Verification items for the finished model (mm, model axes). A direction names the side the tool comes from. Give positions to 0.01 mm unless a question says otherwise; leave off trailing zeros. Loops run counter-clockwise (first coordinate to the right, second up) from the corner with the lowest first, then second, coordinate; pieces in that order, holes last. Notation, with made-up numbers: M 15,73.5 L 53,73.5 A21 cw 53,112.5 Z; hole C -25.5,72.5 d10. An arc over 180 degrees is marked long. Put each result on its own line as item: value. Start each with the question number.
from build123d import *

# Parameters (mm, degrees)
SKETCH1_R           = 1.375
BOSS_EXTRUDE1_DEPTH = 6
BOSS_EXTRUDE2_START = -13.125
SKETCH9_W           = 3.5
SKETCH9_H           = 3
BOSS_EXTRUDE2_DEPTH = 7.26
BOSS_EXTRUDE3_START = -26.75
SKETCH10_W          = 3
SKETCH10_H          = 3
BOSS_EXTRUDE3_DEPTH = 23.25
SKETCH11_W          = 3
SKETCH11_H          = 3
BOSS_EXTRUDE4_DEPTH = 5
FILLET1_R           = 2.5
FILLET2_R           = 1


with BuildPart() as part:
    # Sketch1 → Boss-Extrude1 (new body)
    with BuildSketch(Plane(origin=(0, 0, 0), x_dir=(0, 1, 0), z_dir=(0, 0, 1))):
        with BuildLine():
            Line((0, 2.875), (7, 2.875))
            Line((7, 2.875), (7, -2.875))
            Line((7, -2.875), (0, -2.875))
            ThreePointArc((0, -2.875), (-2.875, 0), (0, 2.875))
        make_face()
        with Locations(Location((0, 0, 0), (0, 0, 270))):
            Circle(SKETCH1_R, mode=Mode.SUBTRACT)
    extrude(amount=BOSS_EXTRUDE1_DEPTH)

    # Sketch2 → Loft1 section 0
    with BuildSketch(Plane(origin=(0, 0, 0), x_dir=(1, 0, 0), z_dir=(0, 0, -1))):
        with BuildLine():
            Line((0.875, -7), (-2.875, -7))
            Line((-2.875, -7), (-2.875, -3.5))
            Line((-2.875, -3.5), (0.875, -3.5))
            Line((0.875, -3.5), (0.875, -7))
        make_face()
    # Sketch8 → Loft1 section 1
    with BuildSketch(Plane(origin=(0, 0, -37.5), x_dir=(-1, 0, 0), z_dir=(0, 0, -1))):
        with BuildLine():
            Line((2.375, 3.5), (2.375, 7))
            Line((2.375, 7), (6.125, 7))
            Line((6.125, 7), (6.125, 3.5))
            Line((6.125, 3.5), (2.375, 3.5))
        make_face()
    loft()

    # Sketch9 → Boss-Extrude2 (add)
    with BuildSketch(Plane.YZ.offset(BOSS_EXTRUDE2_START)):
        with Locations((5.25, -36)):
            Rectangle(SKETCH9_W, SKETCH9_H)
    extrude(amount=BOSS_EXTRUDE2_DEPTH)

    # Sketch10 → Boss-Extrude3 (add)
    with BuildSketch(Plane(origin=(0, 7, 0), x_dir=(-1, 0, 0), z_dir=(0, 1, 0)).offset(BOSS_EXTRUDE3_START)):
        with Locations((11.625, -36)):
            Rectangle(SKETCH10_W, SKETCH10_H)
    extrude(amount=BOSS_EXTRUDE3_DEPTH)

    # Sketch11 → Boss-Extrude4 (add)
    with BuildSketch(Plane.XY.offset(-34.5)):
        with Locations((-11.625, -18.25)):
            Rectangle(SKETCH11_W, SKETCH11_H)
    extrude(amount=BOSS_EXTRUDE4_DEPTH)

    # Fillet1
    # the kernel refuses this fillet: 2.5 mm, written as the material it adds along each edge
    with BuildSketch(Plane(origin=(-10.125, 3.5, -37.5), x_dir=(1, 0, 0), z_dir=(0, 0, 1))) as fillet1_piece_1:
        with BuildLine():
            CenterArc((FILLET1_R, -FILLET1_R), FILLET1_R, 90, 90)
            Line((0, -FILLET1_R), (0, 0))
            Line((0, 0), (FILLET1_R, 0))
        make_face()
    extrude(amount=3)
    with BuildSketch(Plane(origin=(0.875, 3.5, 0), x_dir=(-0.08634300732914678, 0, -0.9962654691824658), z_dir=(0, 1, 0))) as fillet1_piece_2:
        with BuildLine():
            CenterArc((2.275267243, -2.5), FILLET1_R, 90, 78.288278187)
            Line((-0.172686015, -1.992530938), (0, 0))
            Line((0, 0), (2.275267243, 0))
        make_face()
    extrude(amount=3.5)
    # the kernel refuses this fillet: 2.5 mm, written as the material it takes off along each edge
    with BuildSketch(Plane(origin=(-2.375, -2.231761645, -37.5), x_dir=(-1, 0, 0), z_dir=(0, 1, 0))) as fillet1_2_piece_1:
        with BuildLine():
            CenterArc((FILLET1_R * 0.917081863151, FILLET1_R), FILLET1_R, 184.953257478, 85.046742522)
            Line((-FILLET1_R * 0.0791836060315, FILLET1_R * 0.913656992671), (0, 0))
            Line((0, 0), (FILLET1_R * 0.917081863151, 0))
        make_face()
    extrude(amount=14.963523289, mode=Mode.SUBTRACT)
    with BuildSketch(Plane(origin=(-13.125, 7, -43.75), x_dir=(0, -1, 0), z_dir=(0, 0, 1))) as fillet1_2_piece_2:
        with BuildLine():
            CenterArc((FILLET1_R, FILLET1_R), FILLET1_R, 180, 90)
            Line((0, FILLET1_R), (0, 0))
            Line((0, 0), (FILLET1_R, 0))
        make_face()
    extrude(amount=15.5, mode=Mode.SUBTRACT)
    with BuildSketch(Plane(origin=(-19.375, -19.75, -37.5), x_dir=(0, 0, 1), z_dir=(1, 0, 0))) as fillet1_2_piece_3:
        with BuildLine():
            CenterArc((FILLET1_R, -FILLET1_R), FILLET1_R, 90, 90)
            Line((0, -FILLET1_R), (0, 0))
            Line((0, 0), (FILLET1_R, 0))
        make_face()
    extrude(amount=15.5, mode=Mode.SUBTRACT)

    # Fillet2
    fillet2_edges = [part.edges().sort_by_distance(p)[0] for p in [
        (0, 7, 6),
        (-5.865, 5.25, -34.5),
        (-11.625, -16.75, -34.5),
        (-11.625, -16.75, -29.5),
        (-13.125, -18.25, -29.5),
        (-11.625, -19.75, -29.5),
        (-10.125, -18.25, -29.5),
    ]]
    fillet(fillet2_edges, radius=FILLET2_R)


solid = part.part
Q1. Cross-section at A-A, the plane x = 0. Record the boundary of the cut face in (y, z) (3 decimals), then the cut area to 3 significant figures.
Q2. Scan lines: L1, parallel to Y at x = 0, z = 3.85 (3 decimals); L2, parallel to Z at x = -12, y = 2.75; L3, parallel to Y at x = -3.75, z = -22. Record each from-to range of solid material in increasing order.
Q3. Go/stop test with flat-tipped pins: pin 1 (6.5 mm diameter, centred on x = 0, y = 1.5, fed in from -Z); pin 2 (3 mm diameter, centred on y = 3, z = -22, fed in from -X); pin 3 (7 mm diameter, centred on x = -9, y = -2, fed in from +Z). Record where each tip stops, or that it passes through.
Q4. Cross-section at C-C, the plane z = -12. Record the boundary of the cut face in (x, y) (3 decimals), then the cut area to 3 significant figures.
Q5. Cross-section at B-B, the plane y = -10.25. Record the boundary of the cut face in (x, z) (3 decimals), then the cut area to 3 significant figures.
Q6. Release check for a two-part mould opening along Y. For faces 1 (the face through (-0.3, -1.34, 2.96)), 2 (the face through (0, 3, 6)), 3 (the face through (-3, 7, -17)) record: pulls with the +Y half, pulls with the -Y half, needs draft (parallel to the pull), parting line crosses it, or undercut.
Q7. Set-up check for faces 4 (the face through (-2.875, 3, 3)), 5 (the face through (0, 2, 0)), 6 (the face through (-10.125, -10, -36)), 7 (the face through (-11, -2, -34.5)): record each of +Z, -Z, +X, -X, +Y, -Y from which the full face is reachable in a straight line by a thin tool's end or side.
Ans:
1. outline: M -2.875,0 L -1.375,0 L -1.375,6 L -2.875,6 Z; M 1.375,0 L 3.5,0 L 3.5,-10.096 L 7,-10.096 L 7,5 A1 ccw 6,6 L 1.375,6 Z
1. area: 77.9 mm^2
2. L1: y = -2.875 to -1.375, 1.375 to 7
2. L2: z = -37.5 to -34.5
2. L3: y = 3.5 to 7
3. pin 1: stops at z = -36.35
3. pin 2: stops at x = -4.9
3. pin 3: stops at z = -34.5
4. outline: M -3.915,3.5 L -0.165,3.5 L -0.165,7 L -3.915,7 Z
4. area: 13.1 mm^2
5. outline: M -13.125,-37.5 L -10.125,-37.5 L -10.125,-34.5 L -13.125,-34.5 Z
5. area: 9.00 mm^2
6. face 1: undercut
6. face 2: needs draft
6. face 3: pulls with the +Y half
7. face 4: +Z, -X, +Y, -Y
7. face 5: -Z, +X, -X, -Y
7. face 6: +Z, -Z, +X, -Y
7. face 7: +Z, -X, +Y
